Verification items for the finished model (mm, model axes). Face numbers are marked on the shaded views. Coordinates: 2 decimals unless noted, no trailing zeros. Order: outer loops, then holes, each group sorted by start corner. A loop starts at its lowest first (then second) coordinate and runs counter-clockwise, first axis right, second up.
Q1. Thickness scan on line 1 (X direction, y = 0, z = -2.35) (3 decimals); line 2 (X direction, y = 0, z = -3.1). Record the ranges inside material, lowest first.
Q2. Draft check along X on the marked faces 1, 2 and 3. Enter one of: pulls with the +X half, pulls with the -X half, needs draft (parallel to the pull), parting line crosses it, or undercut.
Q3. Depth check by flat-ended pin: P1, Ø5.5, axis at x = -1, y = -1.5, coming from the -Z side; P2, Ø8, axis at x = -6.5, y = -19, coming from the +Z side; P3, Ø0.9, axis at x = 0, z = -8, coming from the -Y side. Enter the tip coordinate at first touch or a pass-through.
Q4. Cross-section at A-A, the plane z = -5.5. Record the boundary of the cut face in (x, y).
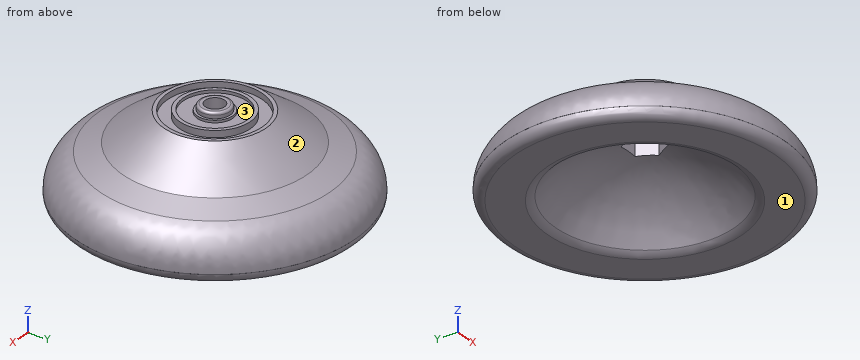
from build123d import *

# Parameters (mm, degrees)
F2_R     = 25
F3_R     = 8
F4_R     = 0.5
F5_R     = 2
F8_DEPTH = 3.5


# Not quite as in the source:
# - a feature names something its author has since deleted; it is built from what else it names


with BuildPart() as f1:
    # F0 (on Front) → F1 (revolve)
    with BuildSketch(Plane.XZ):
        Polygon((3.175, -1.2), (2, -1.2), (2, -9), (12.8490433491, -10.9498299199), (19.1417375121, -20), (29, -20), (29, -12.5), (19.1417375121, -8.7112029778), (10.6, -2.5), (9.85, -2.5), (9.85, -3.7), (7.35, -3.7), (7.35, -2.3), (6.6, -2.3), (6.6, -2.9), (3.675, -2.9), (3.675, -2.4), (3.175, -2.4), align=None)
    revolve(axis=Axis((0, 0, -7.3547498323), (0, 0, -1)))

    # F2
    f2_edges = [f1.edges().sort_by_distance(p)[0] for p in [
        (-12.849043, 0, -10.94983),
    ]]
    fillet(f2_edges, radius=F2_R)

    # F3
    f3_edges = [f1.edges().sort_by_distance(p)[0] for p in [
        (-29, 0, -12.5),
    ]]
    fillet(f3_edges, radius=F3_R)

    # F4
    f4_edges = [f1.edges().sort_by_distance(p)[0] for p in [
        (-3.175, 0, -1.2),
    ]]
    fillet(f4_edges, radius=F4_R)

    # F5
    f5_edges = [f1.edges().sort_by_distance(p)[0] for p in [
        (-29, 0, -20),
        (-19.141738, 0, -20),
    ]]
    fillet(f5_edges, radius=F5_R)

    # F7 (on offset) → F8 (cut)
    with BuildSketch(Plane.XY.offset(-6.5)):
        Polygon((2.0207259422, -3.5), (4.0414518843, 0), (2.0207259422, 3.5), (-2.0207259422, 3.5), (-4.0414518843, 0), (-2.0207259422, -3.5), align=None)
    extrude(amount=-F8_DEPTH, mode=Mode.SUBTRACT)


solid = f1.part
Check values:
1. line 1: x = -7.35 to -6.6, -3.175 to -2, 2 to 3.175, 6.6 to 7.35
1. line 2: x = -11.43 to -9.85, -7.35 to -2, 2 to 7.35, 9.85 to 11.43
2. face 1: needs draft
2. face 2: parting line crosses it
2. face 3: undercut
3. P1: stops at z = -9.54
3. P2: stops at z = -6.49
3. P3: stops at y = -18.78
4. outline: circle Ø29.45 at (0, 0); hole circle Ø4 at (0, 0)
